```python
from build123d import *

# Parameters (mm, degrees)
F0_W     = 304.8
F0_H     = 25.4
F1_DEPTH = 9.525


with BuildPart() as f1:
    # F0 (on Front) → F1 (new body)
    with BuildSketch(Plane.XZ):
        with Locations((474.0515406549, 97.119426218)):
            Rectangle(F0_W, F0_H)
        Polygon((315.3015375137, 52.669426218), (321.6515406549, 52.669426218), (321.6515406549, 84.419426218), (321.6515406549, 109.819426218), (315.3015375137, 109.819426218), align=None)
        Polygon((365.3527498245, 52.669426218), (626.4515406549, 52.669426218), (626.4515406549, 84.419426218), (321.6515406549, 84.419426218), (321.6515406549, 52.669426218), align=None)
        Polygon((626.4515406549, 84.419426218), (626.4515406549, 52.669426218), (634.3763406549, 66.3955824579), (634.3763406549, 109.819426218), (626.4515406549, 109.819426218), align=None)
        Polygon((634.3763406549, 109.819426218), (634.3763406549, 66.3955824579), (642.3265406549, 80.1657327882), (653.179416568, 98.963465278), align=None)
        Polygon((653.179416568, 98.963465278), (642.3265406549, 80.1657327882), (689.9515406549, 52.669426218), (733.3630443075, 52.669426218), align=None)
        Polygon((642.3265406549, 80.1657327882), (634.3763406549, 66.3955824579), (634.3763406549, 52.669426218), (689.9515406549, 52.669426218), align=None)
        Polygon((634.3763406549, 66.3955824579), (626.4515406549, 52.669426218), (634.3763406549, 52.669426218), align=None)
        Polygon((802.4279027039, -48.930573782), (634.3763406549, 48.0940408048), (634.3763406549, -55.7142719626), (807.9667468622, -55.7142719626), (836.2473392138, -6.7308491415), (829.155778617, -2.636534722), (818.3029027039, -21.4342672118), align=None)
        Polygon((634.3763406549, 52.669426218), (634.3763406549, 48.0940408048), (802.4279027039, -48.930573782), (818.3029027039, -21.4342672118), (689.9515406549, 52.669426218), align=None)
        Polygon((733.3630443075, 52.669426218), (689.9515406549, 52.669426218), (818.3029027039, -21.4342672118), (829.155778617, -2.636534722), align=None)
        Polygon((836.2473392138, -6.7308491415), (807.9667468622, -55.7142719626), (824.2119550705, -55.7142719626), (854.6004848789, -55.7142719626), (871.1648442681, -27.0239599059), (848.3022022869, -13.73680994), align=None)
        Polygon((871.1648442681, -27.0239599059), (854.6004848789, -55.7142719626), (878.8170780003, -55.7142719626), (878.8170780003, -31.4712314529), align=None)
    extrude(amount=F1_DEPTH)


solid = f1.part
```
Check sheet for the modelled part. Datum: model origin and axes. Units: mm. A direction names the side the tool comes from. Coordinates: 2 decimals unless noted, no trailing zeros. Order: outer loops, then holes, each group sorted by start corner. A loop starts at its lowest first (then second) coordinate and runs counter-clockwise, first axis right, second up. Notation, with made-up numbers: M -17.5,-18.75 L 4.5,-18.75 A30 cw 4.5,9.25 Z; hole C -18.75,83.5 d5. An arc over 180 degrees is marked long. Write each question's results on one line, items separated by ' | '. Start each with the question number.
1. Cross-section at C-C on z = 72. Record the cut outline in (x, y) (1 decimal), and give its area (3 significant figures).
2. Cross-section at B-B on x = 520. Record the cut outline in (y, z) (3 decimals), and give its area (3 significant figures).
3. Material ranges on probe 1 along X at (y, z) = (-0.75, -47); probe 2 along Z at (x, y) = (508.5, -5.5); probe 3 along X at (y, z) = (-7.75, -4), recorded low to high.
4. Mould release check, pull along Y, two halves, no side actions. Record for faces 1 (the face through (593, -9.525, 65)), 2 (the face through (473, -5, 52.669)), 3 (the face through (593, 0, 65)): +Y half, -Y half, draft (parallel to the pull), parting line (faces both ways), or undercut.
5. Access from +Z, -Z, +X, -X, +Y, -Y to the whole of each face (thin tool, end or side, straight path). Record for faces 4 (the face through (878.817, -5, -44)), 5 (the face through (634.376, -5, -1)).
6. Cross-section at A-A on y = -3. Record the cut outline in (x, z).
7. Go/stop test with flat-tipped pins: P1, Ø4, axis at y = -2.5, z = 10, coming from the +X side; P2, Ø4, axis at y = -2.5, z = 43, coming from the -X side. Record where each tip stops, or that it passes through.
Checks:
1) outline: M 315.3,-9.5 L 699.9,-9.5 L 699.9,0 L 315.3,0 Z | area: 3,660 mm²
2) outline: M -9.525,52.669 L 0,52.669 L 0,109.819 L -9.525,109.819 Z | area: 544 mm²
3) probe 1: x = 634.38 to 878.82 | probe 2: z = 52.67 to 109.82 | probe 3: x = 634.38 to 831.52
4) face 1: -Y half | face 2: draft | face 3: +Y half
5) face 4: +Z, -Z, +X, +Y, -Y | face 5: -Z, -X, +Y, -Y
6) outline: M 315.3,52.67 L 634.38,52.67 L 634.38,-55.71 L 878.82,-55.71 L 878.82,-31.47 L 836.25,-6.73 L 634.38,109.82 L 315.3,109.82 Z
7) P1: stops at x = 810.73 | P2: stops at x = 634.38
